```python
from build123d import *

# Parameters (mm, degrees)
SKETCH1_R             = 2.5
BOSS_EXTRUDE1_DEPTH   = 16
CHAMFER1_SIZE         = 0.3
CHAMFER1_SIZE2        = 0.519615242
CHAMFER1_PART_2_SIZE  = 0.3
CHAMFER1_PART_2_SIZE2 = 0.519615242


with BuildPart() as part:
    # Sketch1 → Boss-Extrude1 (new body)
    with BuildSketch(Plane(origin=(0, 0, 0), x_dir=(1, 0, 0), z_dir=(0, 1, 0))):
        Circle(SKETCH1_R)
    extrude(amount=BOSS_EXTRUDE1_DEPTH)

    # Chamfer1
    chamfer1_edges = [part.edges().sort_by_distance(p)[0] for p in [
        (-2.5, 0, 0),
    ]]
    chamfer1_side = [part.faces().sort_by_distance(p)[0] for p in [
        (0, 0, 0),
    ]]
    chamfer(chamfer1_edges, length=CHAMFER1_SIZE, length2=CHAMFER1_SIZE2, reference=chamfer1_side[0])

    # Chamfer1 part 2
    chamfer1_part_2_edges = [part.edges().sort_by_distance(p)[0] for p in [
        (-2.5, 16, 0),
    ]]
    chamfer1_part_2_side = [part.faces().sort_by_distance(p)[0] for p in [
        (-2.5, 8, 0),
    ]]
    chamfer(chamfer1_part_2_edges, length=CHAMFER1_PART_2_SIZE, length2=CHAMFER1_PART_2_SIZE2, reference=chamfer1_part_2_side[0])


solid = part.part
```
Model file for the job. Use its own axes, mm. Give positions to 0.01 mm unless a question says otherwise; leave off trailing zeros. Loops run counter-clockwise (first coordinate to the right, second up) from the corner with the lowest first, then second, coordinate; pieces in that order, holes last. Notation, with made-up numbers: (41.5, -40) - (100.5, -40) arc R16 ccw to (100.5, -23) - close; hole circle Ø6 at (28, 28.5). An arc over 180 degrees is marked (long way). One line per item, written item: value. Start each with the question number.
1. Probe L1, parallel to X at y = 11, z = 0.1; L2, parallel to Z at x = 0.65, y = 11.25; L3, parallel to Z at x = -0.4, y = 15. List the from-to ranges inside material, lowest first. Write a range as from..to.
2. Slice it at A-A (y = 1). List the corners of the cut face in (x, z), plus the area to 3 significant figures.
3. Pin check, flat tips, straight feed: pin 1 (2 mm diameter, centred on x = 1.5, y = 11.5, fed in from -Z); pin 2 (3 mm diameter, centred on x = 2, y = 10, fed in from +Z); pin 3 (2 mm diameter, centred on x = 1.5, z = -0.5, fed in from -Y). Stop position of each tip, or through.
Solution:
1. L1: x = -2.5..2.5
1. L2: z = -2.41..2.41
1. L3: z = -2.47..2.47
2. outline: circle Ø5 at (0, 0)
2. area: 19.6 mm^2
3. pin 1: stops at z = -2.45
3. pin 2: stops at z = 2.45
3. pin 3: stops at y = 0
